The model under review builds one solid part; all positions refer to its coordinate system, in mm. Face numbers are marked on the shaded views. Coordinates: 2 decimals unless noted, no trailing zeros. Loops run counter-clockwise (first coordinate to the right, second up) from the corner with the lowest first, then second, coordinate; pieces in that order, holes last. Notation, with made-up numbers: (80, -20) - (100, -20) arc R20 cw to (100, 10) - close; hole circle Ø1 at (12.25, 51.5). An arc over 180 degrees is marked (long way). Use a Markdown table: item, result. Add a question column.
1) The part is to be moulded in two halves that separate along X. For the marked faces 1, 2 and 3, say which applies: pulls with the +X half, pulls with the -X half, needs draft (parallel to the pull), parting line crosses it, or undercut.
2) Add section A-A, the plane x = 26. Give the boundary of the cut face in (y, z).
3) Add section B-B, the plane y = 0. Give the boundary of the cut face in (x, z).
4) To check wall thickness, follow L1, parallel to Y at x = 0, z = 160.05; L2, parallel to Y at x = 0, z = 120; L3, parallel to Z at x = 146.5, y = 42. State the ranges of each line that lie inside material, in increasing order. Write a range as [from, to].
5) Clearance check with flat-ended pins moving along their axes: pin 1 (10 mm diameter, centred on x = 109, y = 149.5, fed in from -Z); pin 2 (13 mm diameter, centred on x = -122.85, y = -169.08, fed in from -Z); pin 3 (1.5 mm diameter, centred on y = -73, z = 129, fed in from +X); pin 4 (7 mm diameter, centred on x = 198.77, y = 64.58, fed in from +Z). State where each tip first meets the part, or that it passes through.
6) Add section C-C, the plane z = 23. Give the boundary of the cut face in (x, y), and give its area (3 significant figures).
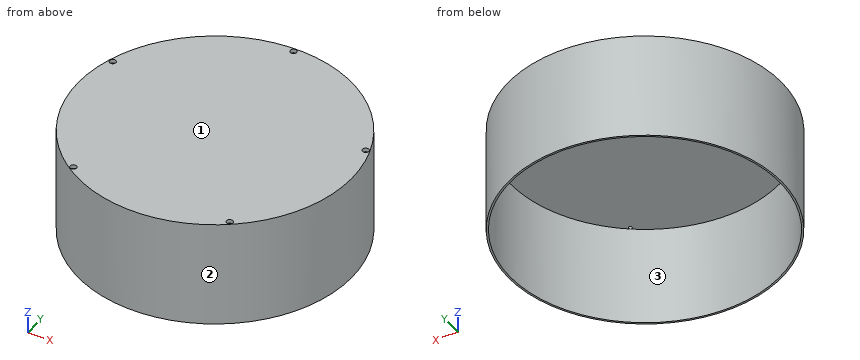
```python
from build123d import *

# Parameters (mm, degrees)
SKETCH1_R              = 215
BODY_DEPTH             = 167
SKETCH2_R              = 212
CAVITY_DEPTH           = 157
SKETCH3_R              = 2.75
ROD_HOLES_DEPTH        = 10
SKETCH4_R              = 5
NUT_COUNTERBORES_DEPTH = 6


with BuildPart() as part:
    # Sketch1 → Body (new body)
    with BuildSketch(Plane.XY):
        with Locations(Location((0, 0, 0), (0, 0, 180))):
            Circle(SKETCH1_R)
    extrude(amount=BODY_DEPTH)

    # Sketch2 → Cavity (cut)
    with BuildSketch(Plane.XY):
        Circle(SKETCH2_R)
    extrude(amount=CAVITY_DEPTH, mode=Mode.SUBTRACT)

    # Sketch3 → Rod_holes (cut)
    with BuildSketch(Plane.XY.offset(157)):
        with Locations((198.770811906, 64.584551824)):
            Circle(SKETCH3_R)
        with Locations((0, 209)):
            Circle(SKETCH3_R)
        with Locations((-198.770811906, 64.584551824)):
            Circle(SKETCH3_R)
        with Locations((-122.847117729, -169.084551824)):
            Circle(SKETCH3_R)
        with Locations((122.847117729, -169.084551824)):
            Circle(SKETCH3_R)
    extrude(amount=ROD_HOLES_DEPTH, mode=Mode.SUBTRACT)

    # Sketch4 → Nut_counterbores (cut)
    with BuildSketch(Plane.XY.offset(161)):
        with Locations((198.770811906, 64.584551824)):
            Circle(SKETCH4_R)
        with Locations((0, 209)):
            Circle(SKETCH4_R)
        with Locations((-198.770811906, 64.584551824)):
            Circle(SKETCH4_R)
        with Locations((-122.847117729, -169.084551824)):
            Circle(SKETCH4_R)
        with Locations((122.847117729, -169.084551824)):
            Circle(SKETCH4_R)
    extrude(amount=NUT_COUNTERBORES_DEPTH, mode=Mode.SUBTRACT)


solid = part.part
```
From the geometry:
| question | item | result |
|---|---|---|
| 1 | face 1 | needs draft |
| 1 | face 2 | parting line crosses it |
| 1 | face 3 | undercut |
| 2 | outline | (-213.42, 0) - (-210.4, 0) - (-210.4, 157) - (210.4, 157) - (210.4, 0) - (213.42, 0) - (213.42, 167) - (-213.42, 167) - close |
| 3 | outline | (-215, 0) - (-212, 0) - (-212, 157) - (212, 157) - (212, 0) - (215, 0) - (215, 167) - (-215, 167) - close |
| 4 | L1 | y = [-215, 206.25], [211.75, 215] |
| 4 | L2 | y = [-215, -212], [212, 215] |
| 4 | L3 | z = [157, 167] |
| 5 | pin 1 | stops at z = 157 |
| 5 | pin 2 | stops at z = 0 |
| 5 | pin 3 | stops at x = 202.5 |
| 5 | pin 4 | stops at z = 161 |
| 6 | outline | circle Ø430 at (0, 0); hole circle Ø424 at (0, 0) |
| 6 | area | 4,020 mm^2 |
